Autodesk Inventor part; units mm, degrees
ref_plane "YZ Plane" through (0, 0, 0) normal (1, 0, 0) x (0, 1, 0)
ref_plane "XZ Plane" through (0, 0, 0) normal (0, 1, 0) x (-1, 0, 0)
ref_plane "XY Plane" through (0, 0, 0) normal (0, 0, 1) x (1, 0, 0)
sketch "Sketch1" plane through (0, 0, 0) normal (0, 1, 0) x (-1, 0, 0)
  circle A0 centre (27.2044, 12.7622) radius 2.075
  arc A1 (27.2044, 9.5122) -> (27.2044, 16.0122) centre (27.2044, 12.7622) ccw
  circle A2 centre (-1.2956, 12.7622) radius 2.075
  arc A3 (-1.2956, 16.0122) -> (-1.2956, 9.5122) centre (-1.2956, 12.7622) ccw
  line L0 (27.2044, 16.0122) -> (-1.2956, 16.0122)
  line L1 (27.2044, 9.5122) -> (-1.2956, 9.5122)
  point P0 (0, 0)
  dimension "d1" = 4.15
  dimension "d4" = 4.15
extrude "Extrusion1" add sketch "Sketch1" along normal blind 5
properties part number "innerBar"
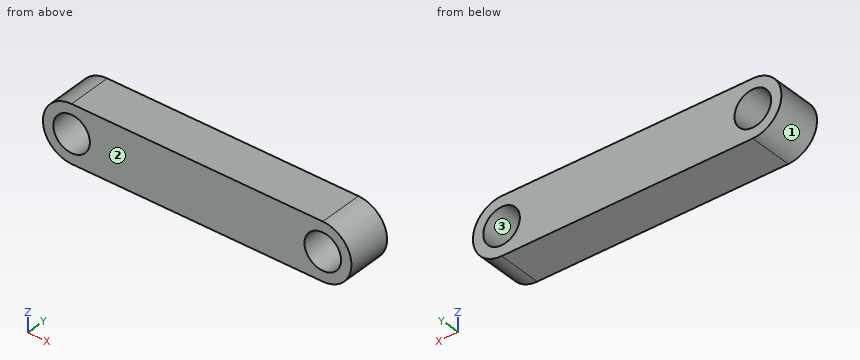
Check sheet for the modelled part. Datum: model origin and axes. Units: mm. Face numbers are marked on the shaded views. Coordinates: 2 decimals unless noted, no trailing zeros. Write each loop counter-clockwise with the first axis right and the second up, starting at its lowest first coordinate (ties: lowest second). Pieces come first, ordered by that corner, then holes. Notation, with made-up numbers: M -32,0.25 L 13,0.25 A30 cw 13,23.25 Z; hole C 47,26.5 d1. An arc over 180 degrees is marked long. Answer as CSV lines item,"result".
Q1. Cross-section at A-A (z = 14). Record the boundary of the cut face in (x, y), then the cut area to 3 significant figures.
Check result:
outline,"M -30.21,0 L -28.87,0 L -28.87,5 L -30.21,5 Z; M -25.54,0 L -0.37,0 L -0.37,5 L -25.54,5 Z; M 2.96,0 L 4.3,0 L 4.3,5 L 2.96,5 Z"
area,"139 mm^2"
Q2. Go/stop test with a flat-tipped pin: pin 1 (2 mm diameter, centred on y = 1.5, z = 11, fed in from +X). Record where the tip stops, or that it passes through.
Check result:
pin 1,"x = 4.45"
Q3. Material ranges on probe 1 along X at (y, z) = (0.65, 12.5) (3 decimals); probe 2 along X at (y, z) = (4.1, 13.5) (3 decimals); probe 3 along Z at (x, y) = (-28, 2.2), recorded low to high. Write a range as from..to.
Check result:
probe 1,"-30.444..-29.263, -25.146..-0.763, 3.354..4.535"
probe 2,"-30.37..-29.144, -25.265..-0.644, 3.235..4.461"
probe 3,"9.61..10.85, 14.68..15.91"
Q4. Cross-section at C-C (z = 11.75). Record the boundary of the cut face in (x, y).
Check result:
outline,"M -30.29,0 L -29.02,0 L -29.02,5 L -30.29,5 Z; M -25.39,0 L -0.52,0 L -0.52,5 L -25.39,5 Z; M 3.11,0 L 4.38,0 L 4.38,5 L 3.11,5 Z"
Q5. Mould release check, pull along X, two halves, no side actions. Record for the marked faces 1, 2 and 3: released by +X, released by -X, zero draft, split by the parting line, or undercut.
Check result:
face 1,"released by -X"
face 2,"zero draft"
face 3,"undercut"
Q6. Cross-section at D-D (z = 10). Record the boundary of the cut face in (x, y), then the cut area to 3 significant figures.
Check result:
outline,"M -28.92,0 L 3.01,0 L 3.01,5 L -28.92,5 Z"
area,"160 mm^2"
Q7. Cross-section at B-B (y = 2.75). Record the boundary of the cut face in (x, z) (3 decimals), then the cut area to 3 significant figures.
Check result:
outline,"M -27.204,9.512 L 1.296,9.512 A3.25 ccw 1.296,16.012 L -27.204,16.012 A3.25 ccw Z; hole C -27.204,12.762 d4.15; hole C 1.296,12.762 d4.15"
area,"191 mm^2"
